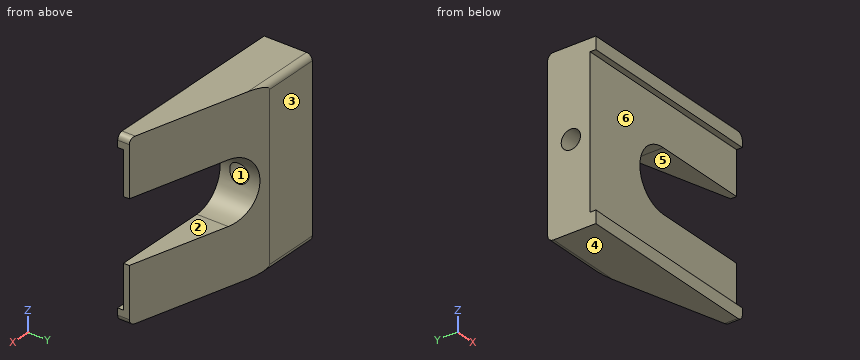
Autodesk Inventor part; units mm, degrees
ref_plane "YZ Plane" through (0, 0, 0) normal (1, 0, 0) x (0, 1, 0)
ref_plane "XZ Plane" through (0, 0, 0) normal (0, 1, 0) x (-1, 0, 0)
ref_plane "XY Plane" through (0, 0, 0) normal (0, 0, 1) x (1, 0, 0)
sketch "Sketch1" plane through (0, 0, 0) normal (0, 1, 0) x (-1, 0, 0)
  arc A0 (0, -16) -> (0, 16) centre (0, 0) ccw
  line L0 (0, 16) -> (-50, 16)
  line L1 (-50, 16) -> (-50, -16)
  line L2 (-50, -16) -> (0, -16)
  line L3 (-50, 0) -> (-50, -45)
  line L4 (-50, -45) -> (-50, 45)
  line L5 (-50, 45) -> (50, 45)
  line L6 (50, 45) -> (50, -45)
  line L7 (50, -45) -> (-50, -45)
  dimension "d1" = 32
  dimension "d2" = 50
  dimension "d3" = 45
  dimension "d4" = 90
  dimension "d5" = 100
extrude "Extrusion1" add sketch "Sketch1" along normal blind 25 contours A0 L0 L4 L5 L6 L7 L3 L2
sketch "Sketch2" plane through (-50, 0, 45) normal (0, 0, 1) x (1, 0, 0)
  line L0 (0, 0) -> (100, 0)
  line L1 (50, 0) -> (100, 0)
  line L2 (100, 0) -> (100, 6)
  line L3 (100, 0) -> (100, 25)
  line L4 (0, 0) -> (0, 25)
  line L5 (0, 25) -> (29.091, 25)
  line L6 (0, 25) -> (100, 25)
  line L7 (29.091, 25) -> (100, 6)
  line L8 (29.091, 25) -> (100, 25)
  line L9 (100, 25) -> (100, 6)
  dimension "d8" = 6
extrude "Extrusion2" cut sketch "Sketch2" against normal through all contours L6 L3 L7
sketch "Sketch3" plane through (50, 0, 45) normal (1, 0, 0) x (0, 0, -1)
  line L0 (45, 0) -> (83.5, 0)
  line L1 (90, 0) -> (0, 0)
  line L2 (45, 0) -> (6.5, 0)
  line L3 (0, 0) -> (29, 0)
  line L4 (83.5, 0) -> (83.5, 3)
  line L5 (83.5, 3) -> (6.5, 3)
  line L6 (6.5, 0) -> (6.5, 3)
  dimension "d12" = 38.5
  dimension "d13" = 38.5
  dimension "d14" = 3
extrude "Extrusion3" cut sketch "Sketch3" against normal through all
sketch "Sketch4" plane through (-50, 0, 45) normal (-1, 0, 0) x (0, 0, 1)
  line L0 (-45, 0) -> (-45, 13)
  circle A0 centre (-45, 13) radius 5
  dimension "d17" = 13
  dimension "d18" = 10
extrude "Extrusion4" cut sketch "Sketch4" against normal through all
fillet "Fillet1" radius 3 4 edges at (-35.4545, 25, 45) (-35.4545, 25, -45) (50, 3, 45) (50, 3, -45)
equation "\"BendRadius\" = Thickness"
equation "\"BendReliefWidth\" = Thickness"
equation "\"BendReliefDepth\" = 0.5 * Thickness"
equation "\"CornerReliefSize\" = 4 * Thickness"
equation "\"MinimumRemnant\" = 2 * Thickness"
equation "\"TransitionRadius\" = BendRadius"
equation "\"JacobiRadiusSize\" = BendRadius"
equation "\"GapSize\" = Thickness"
properties part number "Sliding Block"
Can you work these out from the model? Positions are in its coordinate system, mm. Face numbers are marked on the shaded views. A direction names the side the tool comes from. Round coordinates to 2 decimals unless told otherwise and drop trailing zeros. Write each loop counter-clockwise with the first axis right and the second up, starting at its lowest first coordinate (ties: lowest second). Pieces come first, ordered by that corner, then holes. Notation, with made-up numbers: (72, 42.5) -> (100, 42.5) arc R34 ccw to (100, 80.5) -> close; hole circle Ø2 at (78, 1.25). An arc over 180 degrees is marked (long way). One line per question, with ' | ' between items. Start each with the question number.
1) Suppose I cut it at B-B on x = 20.5. Write out the boundary of the cut face in (y, z), then the cut area to 3 significant figures.
2) Suppose I cut it at D-D on z = 25.5. Write out the boundary of the cut face in (x, y).
3) I need wall thicknesses on line 1 (Z direction, x = 1.5, y = 9.25); line 2 (Z direction, x = -29, y = 13); line 3 (Y direction, x = -40, z = 0). Which ranges of each line are inside material? Lowest first, please. Write a range as [from, to].
4) On a 3-axis mill with a long thin cutter (end or side, diameter ignored), from which of +Z, -Z, +X, -X, +Y, -Y can I reach the whole of each face in a straight line? I mean the marked faces 4, 5 and 6. Say none if no direction works.
5) If we mould it in two halves opening along Y, with no side actions, what happens to the marked faces 1, 2 and 3? For each: released by +Y, released by -Y, zero draft, split by the parting line, or undercut.
6) Suppose I cut it at A-A on z = 0. Write out the boundary of the cut face in (x, y), then the cut area to 3 significant figures.
7) I'm going to push flat-ended pins straight in: P1, Ø2, axis at x = 36.5, z = -22, coming from the +Y side; P2, Ø23, axis at x = 19.5, z = 12, coming from the -Y side. Where does each tip first touch, or does it pass through?
8) Suppose I cut it at C-C on y = 13. Write out the boundary of the cut face in (x, z).
Return value:
1) outline: (0, -45) -> (13.9, -45) -> (13.9, -16) -> (3, -16) -> (3, -38.5) -> (0, -38.5) -> close; (0, 38.5) -> (3, 38.5) -> (3, 16) -> (13.9, 16) -> (13.9, 45) -> (0, 45) -> close | area: 671 mm2
2) outline: (-50, 3) -> (50, 3) -> (50, 6) -> (-20.91, 25) -> (-50, 25) -> close
3) line 1: z = [-45, -16], [16, 45] | line 2: z = [-45, -5], [5, 45] | line 3: y = [3, 8], [18, 25]
4) face 4: -Z, +X, -X, +Y, -Y | face 5: +X, +Y, -Y | face 6: +X, -X, -Y
5) face 1: undercut | face 2: zero draft | face 3: released by +Y
6) outline: (-50, 3) -> (-16, 3) -> (-16, 8) -> (-50, 8) -> close; (-50, 18) -> (-16, 18) -> (-16, 23.68) -> (-20.91, 25) -> (-50, 25) -> close | area: 405 mm2
7) P1: stops at y = 9.89 | P2: stops at y = 3
8) outline: (-50, -45) -> (23.88, -45) -> (23.88, -16) -> (0, -16) arc R16 cw to (-15.2, -5) -> (-50, -5) -> close; (-50, 5) -> (-15.2, 5) arc R16 cw to (0, 16) -> (23.88, 16) -> (23.88, 45) -> (-50, 45) -> close
